Geometry: final body of the model. Coordinates: model frame, mm. A direction names the side the tool comes from. Give positions to 0.01 mm unless a question says otherwise; leave off trailing zeros. Order: outer loops, then holes, each group sorted by start corner. A loop starts at its lowest first (then second) coordinate and runs counter-clockwise, first axis right, second up. Notation, with made-up numbers: M 33,-3.75 L 46,-3.75 A18 ccw 46,28.25 Z; hole C 73.25,29 d1. An arc over 180 degrees is marked long. Write item = value, one per line. Start each with the question number.
Autodesk Inventor part; units mm, degrees
ref_plane "YZ Plane" through (0, 0, 0) normal (1, 0, 0) x (0, 1, 0)
ref_plane "XZ Plane" through (0, 0, 0) normal (0, 1, 0) x (-1, 0, 0)
ref_plane "XY Plane" through (0, 0, 0) normal (0, 0, 1) x (1, 0, 0)
sketch "Sketch1" plane through (0, 0, 0) normal (0, 1, 0) x (-1, 0, 0)
  line L0 (0, 0) -> (-20.32, 0)
  line L1 (-20.32, 0) -> (-20.32, -15.24)
  line L2 (-20.32, -15.24) -> (0, -15.24)
  line L3 (0, -15.24) -> (0, 0)
  line L4 (-20.32, -7.62) -> (0, -7.62) construction
  circle A0 centre (-17.526, -7.62) radius 1.143
  circle A1 centre (-2.794, -7.62) radius 1.143
  dimension "d0" = 20.32
  dimension "d1" = 15.24
  dimension "d2" = 14.732
  dimension "d3" = 2.794
  dimension "d4" = 2.286
  dimension "d5" = 2.286
extrude "Extrusion1" add sketch "Sketch1" along normal blind 2.032
sketch "Sketch2" plane through (0, 2.032, 0) normal (0, 1, 0) x (1, 0, 0)
  line L0 (0, 15.24) -> (0, 0) construction
  line L1 (0, 7.62) -> (20.32, 7.62) construction
  line L2 (20.32, 0) -> (20.32, 15.24) construction
  line L3 (20.32, 15.24) -> (0, 15.24) construction
  line L4 (10.16, 15.24) -> (10.16, 0) construction
  line L5 (0, 0) -> (20.32, 0) construction
  circle A0 centre (10.16, 7.62) radius 5.08
  dimension "d8" = 10.16
extrude "Extrusion2" add sketch "Sketch2" along normal blind 11.43
properties part number "half_inch_castor"
1) Cut plane C-C (x = 17). Return loops of the section in (y, z).
2) Draft query along Z for faces 1 (the flat face through (10, 0, -8)), 2 (the cylindrical face through (18.43, 1, -6.92)), 3 (the flat face through (10, 1, 0)), 4 (the cylindrical face through (3.042, 1.002, -6.504)). Return one class per face: pulls with the +Z half, pulls with the -Z half, needs draft (parallel to the pull), parting line crosses it, or undercut.
3) Pin query (flat end, axial travel): pin 1 Ø1 at (x, y) = (18, 3) entering from +Z; pin 2 Ø4 at (y, z) = (11, -9.5) entering from -X; pin 3 Ø4 at (x, y) = (8, 5) entering from +Z; pin 4 Ø3 at (y, z) = (11.5, -12) entering from +X. Return the tip coordinate at first contact, or that it passes through.
4) Cut plane A-A (z = -7.62). Return loops of the section in (x, y), plus the area to 3 significant figures.
5) Cut plane D-D (z = -3.75). Return loops of the section in (x, y).
6) Ray query, L1, parallel to Y at x = 4, z = -13.25; L2, parallel to Z at x = 17.5, y = 1; L3, parallel to X at y = 11.25, z = -7.75. Return the intervals inside material, ascending.
7) Cut plane B-B (x = 10.16). Return loops of the section in (y, z), plus the area to 3 significant figures.
8) Access query for faces 5 (the flat face through (10, 1, -15.24)), 6 (the flat face through (10, 2.032, -2)). Directions: +Z, -Z, +X, -X, +Y, -Y. A direction counts if a zero-diameter tool reaches every point of the face in a straight line with its end or side. Return the directions, or none.
Reply:
q1.outline = M 0,-15.24 L 2.03,-15.24 L 2.03,-8.63 L 0,-8.63 Z; M 0,-6.61 L 2.03,-6.61 L 2.03,0 L 0,0 Z
q2.face_1 = needs draft
q2.face_2 = undercut
q2.face_3 = pulls with the +Z half
q2.face_4 = undercut
q3.pin_1 = through
q3.pin_2 = 5.08
q3.pin_3 = -2.54
q3.pin_4 = 14.34
q4.outline = M 0,0 L 1.65,0 L 1.65,2.03 L 0,2.03 Z; M 3.94,0 L 16.38,0 L 16.38,2.03 L 15.24,2.03 L 15.24,13.46 L 5.08,13.46 L 5.08,2.03 L 3.94,2.03 Z; M 18.67,0 L 20.32,0 L 20.32,2.03 L 18.67,2.03 Z
q4.area = 148 mm²
q5.outline = M 0,0 L 20.32,0 L 20.32,2.03 L 13.45,2.03 L 13.45,13.46 L 6.87,13.46 L 6.87,2.03 L 0,2.03 Z
q6.L1 = 0 to 2.03
q6.L2 = -15.24 to -8.76, -6.48 to 0
q6.L3 = 5.08 to 15.24
q7.outline = M 0,-15.24 L 2.03,-15.24 L 2.03,-12.7 L 13.46,-12.7 L 13.46,-2.54 L 2.03,-2.54 L 2.03,0 L 0,0 Z
q7.area = 147 mm²
q8.face_5 = -Z, +X, -X, +Y, -Y
q8.face_6 = +Y
